from build123d import *

# Parameters (mm, degrees)
SPLIT_SADDLE_WITH_37_4_MM_BORE_DEPTH = 14
M4_THROUGH_HOLES_DEPTH               = 44.144988121
M4_THROUGH_HOLES_DEPTH_BACK          = 44.144988121
SKETCH2_R                            = 2.25


with BuildPart() as part:
    # Split saddle with 37.4 mm bore profile → Split saddle with 37.4 mm bore (new body)
    with BuildSketch(Plane.XY):
        with BuildLine():
            Line((-29.5, 7), (29.5, 7))
            Line((29.5, 7), (29.5, 28.2))
            Line((29.5, 28.2), (18.697593428, 28.2))
            ThreePointArc((18.697593428, 28.2), (0, 9.8), (-18.697593428, 28.2))
            Line((-18.697593428, 28.2), (-29.5, 28.2))
            Line((-29.5, 28.2), (-29.5, 7))
        make_face()
    extrude(amount=SPLIT_SADDLE_WITH_37_4_MM_BORE_DEPTH)

    # Sketch2 → M4 through holes (cut, two sides: drawn at the far end of the back side and taken through both)
    with BuildSketch(Plane(origin=(0, 0, 0), x_dir=(1, 0, 0), z_dir=(0, 1, 0)).offset(-M4_THROUGH_HOLES_DEPTH_BACK)):
        with Locations(Location((-24.5, -7, 0), (0, 0, 270))):
            Circle(SKETCH2_R)
        with Locations(Location((24.5, -7, 0), (0, 0, 270))):
            Circle(SKETCH2_R)
    extrude(amount=M4_THROUGH_HOLES_DEPTH + M4_THROUGH_HOLES_DEPTH_BACK, mode=Mode.SUBTRACT)


solid = part.part
Could you check a few things on this model? Use its own coordinates, in mm. Give positions to 0.01 mm unless a question says otherwise; leave off trailing zeros. Order: outer loops, then holes, each group sorted by start corner. A loop starts at its lowest first (then second) coordinate and runs counter-clockwise, first axis right, second up.
Item 1: If we section it at C-C, the plane x = 24.5: Write out the boundary of the cut face in (y, z).
Item 2: I'm going to push flat-ended pins straight in: pin 1 (2 mm diameter, centred on x = 4.5, z = 11.5, fed in from +Y); pin 2 (5 mm diameter, centred on x = 3.5, z = 10.5, fed in from +Y); pin 3 (5 mm diameter, centred on x = 4, y = 9.5, fed in from -Z). Where does each tip first touch, or does it pass through?
Item 3: I need wall thicknesses on line 1 (X direction, y = 18.25, z = 8); line 2 (X direction, y = 16.75, z = 7); line 3 (Z direction, x = 24.5, y = 11). Which ranges of each line are inside material? Lowest first, please.
Item 4: If we section it at D-D, the plane y = 20.5: Write out the boundary of the cut face in (x, z).
Item 5: If we section it at A-A, the plane y = 16: Write out the boundary of the cut face in (x, z), plus the area to 3 significant figures.
Item 6: If we mould it in two halves opening along Z, with no side actions, what happens to faces 1 (the face through (22, 28.2, 7)), 2 (the face through (0, 8, 14)), 3 (the face through (-26.696, 17.452, 6.512)), 4 (the face through (22.304, 17.452, 6.512))? For each: pulls with the +Z half, pulls with the -Z half, needs draft (parallel to the pull), parting line crosses it, or undercut.
Values:
1. outline: (7, 0) - (28.2, 0) - (28.2, 4.75) - (7, 4.75) - close; (7, 9.25) - (28.2, 9.25) - (28.2, 14) - (7, 14) - close
2. pin 1: stops at y = 10.63
2. pin 2: stops at y = 10.79
2. pin 3: stops at z = 0
3. line 1: x = -29.5 to -26.52, -22.48 to -15.64, 15.64 to 22.48, 26.52 to 29.5
3. line 2: x = -29.5 to -26.75, -22.25 to -14.55, 14.55 to 22.25, 26.75 to 29.5
3. line 3: z = 0 to 4.75, 9.25 to 14
4. outline: (-29.5, 0) - (-16.9, 0) - (-16.9, 14) - (-29.5, 14) - close; (16.9, 0) - (29.5, 0) - (29.5, 14) - (16.9, 14) - close; hole circle Ø4.5 at (-24.5, 7); hole circle Ø4.5 at (24.5, 7)
5. outline: (-29.5, 0) - (-13.91, 0) - (-13.91, 14) - (-29.5, 14) - close; (13.91, 0) - (29.5, 0) - (29.5, 14) - (13.91, 14) - close; hole circle Ø4.5 at (-24.5, 7); hole circle Ø4.5 at (24.5, 7)
5. area: 405 mm2
6. face 1: needs draft
6. face 2: pulls with the +Z half
6. face 3: undercut
6. face 4: undercut
